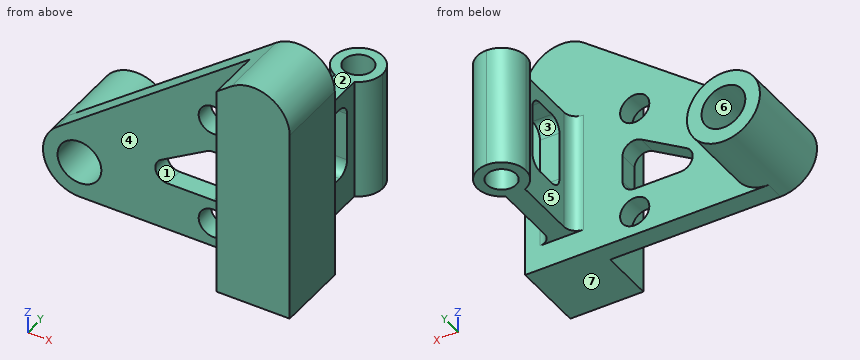
```python
from build123d import *

# Parameters (mm, degrees)
SKETCH1_R           = 15
SKETCH1_R_2         = 9
SKETCH1_R_3         = 6
SKETCH1_W           = 10
SKETCH1_H           = 50
BOSS_EXTRUDE2_DEPTH = 30
SKETCH2_W           = 112.950636881
SKETCH2_H           = 38.744396061
CUT_EXTRUDE1_DEPTH  = 153.151240547
BOSS_EXTRUDE3_START = 30
SKETCH1_3_R         = 15
SKETCH1_3_R_2       = 9
BOSS_EXTRUDE3_DEPTH = 30
SKETCH1_4_W         = 20
SKETCH1_4_H         = 50
BOSS_EXTRUDE4_DEPTH = 50
SKETCH3_R           = 6
CUT_EXTRUDE2_DEPTH  = 140.185416071
FILLET1_R           = 5
CUT_EXTRUDE3_DEPTH  = 8


with BuildPart() as part:
    # Sketch1 → Boss-Extrude2 (new body)
    # profile 1 of 4: a face of its own
    with BuildSketch(Plane(origin=(0, 0, 0), x_dir=(1, 0, 0), z_dir=(0, 1, 0))):
        with Locations((-100, -15)):
            Circle(SKETCH1_R)
        with Locations(Location((-100, -15, 0), (0, 0, 270))):
            Circle(SKETCH1_R_2, mode=Mode.SUBTRACT)
    # profile 2 of 4: a face of its own
    with BuildSketch(Plane(origin=(0, 0, 0), x_dir=(1, 0, 0), z_dir=(0, 1, 0))):
        with BuildLine():
            Line((0, -80), (0, 0))
            Line((0, 0), (-100, 0))
            ThreePointArc((-100, 0), (-89.393398282, -4.393398282), (-85, -15))
            ThreePointArc((-85, -15), (-93.354560745, -28.447607114), (-109.111751614, -26.915367495))
            Line((-109.111751614, -26.915367495), (-24.111751614, -91.915367495))
            ThreePointArc((-24.111751614, -91.915367495), (-8.354560745, -93.447607114), (0, -80))
        make_face()
        with Locations(Location((-45, -55, 0), (0, 0, 270))):
            Circle(SKETCH1_R_3, mode=Mode.SUBTRACT)
        with BuildLine():
            ThreePointArc((-66.381939771, -29.296464422), (-68.64542921, -23.673787745), (-63.824520472, -20))
            Line((-63.824520472, -20), (-45, -20))
            ThreePointArc((-45, -20), (-41.464466094, -21.464466094), (-40, -25))
            Line((-40, -25), (-40, -36.20507171))
            ThreePointArc((-40, -36.20507171), (-42.528876419, -40.551742648), (-47.557419299, -40.501536132))
            Line((-47.557419299, -40.501536132), (-66.381939771, -29.296464422))
        make_face(mode=Mode.SUBTRACT)
        Polygon((-25, -60.395198873), (-25, -10.395198873), (-15, -10.395198873), (-5, -10.395198873), (-5, -60.395198873), (-15, -60.395198873), align=None, mode=Mode.SUBTRACT)
        with Locations(Location((-45, -10, 0), (0, 0, 270))):
            Circle(SKETCH1_R_3, mode=Mode.SUBTRACT)
    # profile 3 of 4: a face of its own
    with BuildSketch(Plane(origin=(0, 0, 0), x_dir=(1, 0, 0), z_dir=(0, 1, 0))):
        with Locations((-10, -35.395198873)):
            Rectangle(SKETCH1_W, SKETCH1_H)
    # profile 4 of 4: a face of its own
    with BuildSketch(Plane(origin=(0, 0, 0), x_dir=(1, 0, 0), z_dir=(0, 1, 0))):
        with Locations((-20, -35.395198873)):
            Rectangle(SKETCH1_W, SKETCH1_H)
    extrude(amount=-BOSS_EXTRUDE2_DEPTH)

    # Sketch2 → Cut-Extrude1 (cut, through all)
    with BuildSketch(Plane(origin=(0, 0, 0), x_dir=(-1, 0, 0), z_dir=(0, 0, -1))):
        with Locations((86.475318441, -27.372198031)):
            Rectangle(SKETCH2_W, SKETCH2_H)
    extrude(amount=-CUT_EXTRUDE1_DEPTH, mode=Mode.SUBTRACT)

    # Sketch1<3> → Boss-Extrude3 (add)
    with BuildSketch(Plane(origin=(0, 0, 0), x_dir=(1, 0, 0), z_dir=(0, 1, 0)).offset(BOSS_EXTRUDE3_START)):
        with Locations(Location((-100, -15, 0), (0, 0, 270))):
            Circle(SKETCH1_3_R)
        with Locations(Location((-100, -15, 0), (0, 0, 270))):
            Circle(SKETCH1_3_R_2, mode=Mode.SUBTRACT)
    extrude(amount=-BOSS_EXTRUDE3_DEPTH)

    # Sketch1<4> → Boss-Extrude4 (add)
    with BuildSketch(Plane(origin=(0, 0, 0), x_dir=(1, 0, 0), z_dir=(0, 1, 0))):
        with Locations((-15, -35.395198873)):
            Rectangle(SKETCH1_4_W, SKETCH1_4_H)
    extrude(amount=BOSS_EXTRUDE4_DEPTH)

    # Sketch3 → Cut-Extrude2 (cut, through all)
    with BuildSketch(Plane.XY.offset(60.395198873)):
        with BuildLine():
            ThreePointArc((-19, 30.83484861), (-23.366600265, 34.522774425), (-25, 40))
            Line((-25, 40), (-25, 0))
            Line((-25, 0), (-19, 0))
            Line((-19, 0), (-19, 30.83484861))
        make_face()
        with BuildLine():
            Line((-5, 0), (-5, 40))
            ThreePointArc((-5, 40), (-6.633399735, 34.522774425), (-11, 30.83484861))
            Line((-11, 30.83484861), (-11, 0))
            Line((-11, 0), (-5, 0))
        make_face()
        with BuildLine():
            Line((-5, 50), (-14.999999965, 50))
            ThreePointArc((-14.999999965, 50), (-7.928932176, 47.0710678), (-5, 40))
            Line((-5, 40), (-5, 50))
        make_face()
        with BuildLine():
            Line((-14.999999965, 50), (-25, 50))
            Line((-25, 50), (-25, 40))
            ThreePointArc((-25, 40), (-22.0710678, 47.071067824), (-14.999999965, 50))
        make_face()
        with Locations((-15, 40)):
            Circle(SKETCH3_R)
    extrude(amount=-CUT_EXTRUDE2_DEPTH, mode=Mode.SUBTRACT)

    # Fillet1
    fillet1_edges = [part.edges().sort_by_distance(p)[0] for p in [
        (-19, 0, 35.395198873),
        (-11, 0, 35.395198873),
    ]]
    fillet(fillet1_edges, radius=FILLET1_R)

    # Sketch4 → Cut-Extrude3 (cut)
    with BuildSketch(Plane(origin=(-11, 0, 0), x_dir=(0, 0, -1), z_dir=(1, 0, 0))):
        with BuildLine():
            Line((-49.395198873, 26), (-29.395198873, 26))
            ThreePointArc((-29.395198873, 26), (-25.859664967, 24.535533906), (-24.395198873, 21))
            Line((-24.395198873, 21), (-24.395198873, 13))
            ThreePointArc((-24.395198873, 13), (-25.859664967, 9.464466094), (-29.395198873, 8))
            Line((-29.395198873, 8), (-49.395198873, 8))
            ThreePointArc((-49.395198873, 8), (-52.930732779, 9.464466094), (-54.395198873, 13))
            Line((-54.395198873, 13), (-54.395198873, 21))
            ThreePointArc((-54.395198873, 21), (-52.930732779, 24.535533906), (-49.395198873, 26))
        make_face()
    extrude(amount=-CUT_EXTRUDE3_DEPTH, mode=Mode.SUBTRACT)


solid = part.part
```
Design review of the part built by this model. Coordinates are the model's own, in mm. Face numbers are marked on the shaded views. A direction names the side the tool comes from. Coordinates: 2 decimals unless noted, no trailing zeros. Loops run counter-clockwise (first coordinate to the right, second up) from the corner with the lowest first, then second, coordinate; pieces in that order, holes last. Notation, with made-up numbers: M 15,-28.75 L 74,-28.75 A26 cw 74,-14.75 Z; hole C -32,8 d5. An arc over 180 degrees is marked long. One line per question, with ' | ' between items.
(1) We need section B-B (z = 45.5). Give the boundary of the cut face in (x, y), and give its area (3 significant figures).
Filled in:
outline: M -84.81,-8 L -30,-8 L -30,-30 L 0,-30 L 0,0 L -6,0 A5 cw -11,5 L -11,8 L -19,8 L -19,5 A5 cw -24,0 L -84.81,0 Z; M -19,26 L -11,26 L -11,30.83 A10 ccw long -19,30.83 Z; hole C -15,40 d12 | area: 1,650 mm^2
(2) We need section C-C (y = 27.5). Give the boundary of the cut face in (x, z).
Filled in:
outline: C -100,15 d30; M -19,10.4 L -11,10.4 L -11,60.4 L -19,60.4 Z; hole C -100,15 d18
(3) We need section D-D (x = -55). Give the boundary of the cut face in (y, z), and give its area (3 significant figures).
Filled in:
outline: M -8,0 L 0,0 L 0,20 L -8,20 Z; M -8,36.07 L 0,36.07 L 0,68.29 L -8,68.29 Z | area: 418 mm^2
(4) Machinability: for the marked faces 1, 2, 3 and 4, which of the approach directions +Z, -Z, +X, -X, +Y, -Y give a long, thin tool a straight path to every point of the face, cutting with its end or side? Answer none if there is none.
Filled in:
face 1: +Y, -Y | face 2: +Z, +X, -X, +Y | face 3: +X, -X | face 4: +Z, -Z, -X, -Y
(5) Draft analysis for pull direction Z (two halves, no side actions). For the marked faces 5, 6 and 7, state which applies: released by +Z, released by -Z, zero draft, split by the parting line, or undercut.
Filled in:
face 5: zero draft | face 6: undercut | face 7: released by -Z
(6) For pin 1 Ø22 at (x, y) = (-17.5, 24) entering from +Z; pin 2 Ø1 at (y, z) = (-17, 77) entering from -X; pin 3 Ø10 at (x, z) = (-62, 19.5) entering from -Y, all flat-tipped, find the tip position at first contact; note any pin that passes through.
Filled in:
pin 1: stops at z = 60.4 | pin 2: stops at x = -30 | pin 3: stops at y = -8
(7) Wall thickness on probe 1 along X at (y, z) = (22, 15); probe 2 along X at (y, z) = (20, 18.5); probe 3 along Y at (x, z) = (-87, 33.5): over which ranges is each line inside the solid? List them lowest first.
Filled in:
probe 1: x = -115 to -109, -91 to -85, -19 to -11 | probe 2: x = -114.59 to -108.29, -91.71 to -85.41, -19 to -11 | probe 3: y = -8 to 0
(8) We need section A-A (y = 19.5). Give the boundary of the cut face in (x, z).
Filled in:
outline: C -100,15 d30; M -19,10.4 L -11,10.4 L -11,24.4 L -19,24.4 Z; M -19,54.4 L -11,54.4 L -11,60.4 L -19,60.4 Z; hole C -100,15 d18
